Autodesk Inventor part; units mm, degrees
ref_plane "YZ Plane" through (0, 0, 0) normal (1, 0, 0) x (0, 1, 0)
ref_plane "XZ Plane" through (0, 0, 0) normal (0, 1, 0) x (-1, 0, 0)
ref_plane "XY Plane" through (0, 0, 0) normal (0, 0, 1) x (1, 0, 0)
sketch "Sketch1" plane through (0, 0, 0) normal (0, 0, 1) x (1, 0, 0)
  circle A0 centre (0, 91.8009) radius 38.1 construction
  circle A1 centre (0, -91.8009) radius 38.1 construction
  line L0 (0, 91.8009) -> (0, -91.8009) construction
  circle A2 centre (-25.4, 0) radius 57.15 construction
  circle A3 centre (0, 91.8009) radius 14.2875
  circle A4 centre (0, -91.8009) radius 14.2875
  circle A5 centre (0, -91.8009) radius 33.3375 construction
  circle A6 centre (0, 91.8009) radius 33.3375 construction
  circle A7 centre (-142.9967, -39.6875) radius 14.3256 construction
  circle A8 centre (0, -91.8009) radius 23.876 construction
  line L1 (-142.9967, -39.6875) -> (0, -91.8009) construction
  circle A9 centre (-142.9967, 39.6875) radius 14.3256 construction
  circle A10 centre (0, 91.8009) radius 23.876 construction
  line L2 (0, 91.8009) -> (-142.9967, 39.6875) construction
  circle A11 centre (-142.9967, 39.6875) radius 39.6875 construction
  circle A12 centre (-142.9967, -39.6875) radius 39.6875 construction
  line L3 (-142.9967, 39.6875) -> (-142.9967, -39.6875) construction
  line L4 (-138.9458, 25.9466) -> (6.7516, 68.8994) construction
  line L5 (-9.5669, 113.6764) -> (-148.7368, 52.8128) construction
  line L6 (-138.9458, -25.9466) -> (6.7516, -68.8994) construction
  circle A13 centre (-142.9967, 39.6875) radius 14.2875
  circle A14 centre (-142.9967, -39.6875) radius 14.2875
  circle A15 centre (-187.9418, -47.625) radius 5.9531 construction
  circle A16 centre (-187.9418, -47.625) radius 9.525
  circle A17 centre (-187.9418, -47.625) radius 17.4625 construction
  circle A18 centre (-187.9418, -47.625) radius 17.4625 construction
  circle A19 centre (-187.9418, -47.625) radius 17.4625 construction
  circle A20 centre (-187.9418, -47.625) radius 17.4625 construction
  circle A21 centre (-187.9418, -47.625) radius 17.4625 construction
  circle A22 centre (-19.05, 0) radius 57.15 construction
  circle A23 centre (-187.9418, -47.625) radius 19.05 construction
  line L7 (-241.3, 101.6) -> (-215.9, 101.6) construction
  line L8 (-215.9, 101.6) -> (-215.9, -101.6) construction
  line L9 (-215.9, -101.6) -> (-241.3, -101.6) construction
  line L10 (-241.3, -101.6) -> (-241.3, 101.6)
  line L11 (-142.9967, -39.6875) -> (-187.9418, -47.625) construction
  line L12 (-77.6563, 63.5) -> (-77.6563, -63.5) construction
  line L13 (-22.4906, -57.0463) -> (2.007, -58.5239)
  arc A24 (2.007, 58.5239) -> (27.142, 111.1581) centre (0, 91.8009) ccw
  arc A25 (-22.4906, 57.0463) -> (-22.4906, -57.0463) centre (-19.05, 0) ccw
  line L14 (2.007, 58.5239) -> (-22.4906, 57.0463)
  arc A26 (27.142, -111.1581) -> (2.007, -58.5239) centre (0, -91.8009) ccw
  arc A27 (3.8774, 143.7787) -> (-0.8591, 145.6978) centre (0, 141.0134) ccw
  circle A28 centre (0, 91.8009) radius 44.45 construction
  line L15 (3.8774, 143.7787) -> (27.142, 111.1581)
  line L16 (-0.8591, 145.6978) -> (-241.3, 101.6)
  arc A29 (-0.8591, -145.6978) -> (3.8774, -143.7787) centre (0, -141.0134) ccw
  line L17 (-241.3, -101.6) -> (-0.8591, -145.6978)
  line L18 (27.142, -111.1581) -> (3.8774, -143.7787)
  circle A30 centre (0, -91.8009) radius 44.45 construction
  line L19 (0, 112.8194) -> (0, 70.7824) construction
  line L20 (-142.9967, 60.706) -> (-142.9967, 18.669) construction
  line L21 (-142.9967, -18.669) -> (-142.9967, -60.706) construction
  line L22 (0, -70.7824) -> (0, -112.8194) construction
  line L23 (-228.6, 50.8) -> (-228.6, -50.8) construction
  line L24 (-187.9418, -15.875) -> (-187.9418, -79.375) construction
  circle A31 centre (-187.9418, -15.875) radius 4.7625 construction
  line L25 (-148.7368, -52.8128) -> (-9.5669, -113.6764) construction
  line L26 (-187.9418, -47.625) -> (-187.9418, -30.1625) construction
  circle A32 centre (-187.9418, -47.625) radius 17.4625 construction
  point P0 (0, 0)
  point P1 (0, 0)
  point P2 (-172.8189, -38.8937)
  point P3 (-203.0648, -38.8938)
  point P4 (-203.0648, -56.3562)
  point P5 (-187.9418, -65.0875)
  point P6 (-215.9, 0)
  point P7 (-228.6, 0)
  point P8 (-228.6, 0)
  point P9 (-228.6, 101.6)
  point P10 (-172.8189, -56.3562)
  dimension "d15" = 34.925
  dimension "d0" = 76.2
  dimension "d1" = 76.2
  dimension "d2" = 114.3
  dimension "d4" = 183.6018
  dimension "d5" = 28.575
  dimension "d6" = 19.05
  dimension "d7" = 28.6512
  dimension "d8" = 47.752
  dimension "d9" = 79.375
  dimension "d10" = 142.9967
  dimension "d11" = 152.1968
  dimension "d12" = 28.575
  dimension "d13" = 11.9062
  dimension "d14" = 19.05
  dimension "d18" = 360
  dimension "d20" = 6.35
  dimension "d21" = 38.1
  dimension "d22" = 25.4
  dimension "d23" = 203.2
  dimension "d24" = 241.3
  dimension "d26" = 127
  dimension "d29" = 9.525
  dimension "d30" = 6.35
  dimension "d32" = 42.037
  dimension "d33" = 42.037
  dimension "d34" = 42.037
  dimension "d35" = 42.037
  dimension "d36" = 25.4
  dimension "d44" = 101.6
  dimension "d45" = 63.5
  dimension "d47" = 9.525
  dimension "d49" = 53.975
extrude "Extrusion1" add sketch "Sketch1" along normal blind 6.35
hole "Hole1" at (-172.8189, -38.8937, 0) at (-187.9418, -30.1625, 0) at (-203.0648, -38.8938, 0) at (-203.0648, -56.3562, 0) at (-187.9418, -65.0875, 0) at (-77.6563, 63.5, 0) at (-77.6563, -63.5, 0) at (0, 112.8194, 0) at (0, 70.7824, 0) at (-142.9967, 60.706, 0) at (-142.9967, 18.669, 0) at (-142.9967, -18.669, 0) at (-142.9967, -60.706, 0) at (0, -70.7824, 0) at (0, -112.8194, 0) at (-228.6, 50.8, 0) at (-228.6, 0, 0) at (-228.6, -50.8, 0) at (-187.9418, -15.875, 0) at (-187.9418, -79.375, 0) at (0, 141.0134, 0) at (0, -141.0134, 0) at (-172.8189, -56.3562, 0) direction (0, 0, 1) diameter 5.1054 end through all
properties part number "GP6-001" material "Polycarbonate, Smoke"
CAD build for the part. Positions are in the model's coordinates, mm. A direction names the side the tool comes from. Give positions to 0.01 mm unless a question says otherwise; leave off trailing zeros. Loops run counter-clockwise (first coordinate to the right, second up) from the corner with the lowest first, then second, coordinate; pieces in that order, holes last. Notation, with made-up numbers: (46, -8) - (97, -8) arc R24 ccw to (97, 31) - close; hole circle Ø1 at (-6, -28). An arc over 180 degrees is marked (long way). Put each result on its own line as item: value.
Q1. Tool access for faces 5 (the face through (-10.07, 57.795, 3.131)), 6 (the face through (-119.396, 123.958, 3.131)): list every direction of +Z, -Z, +X, -X, +Y, -Y with a clear straight run to the whole face (end or side of a thin tool).
Filled in:
face 5: +Z, -Z, +X
face 6: +Z, -Z, -X, +Y
Q2. Mould opens along X. For faces 1 (the face through (-129.799, -34.215, 3.131)), 2 (the face through (-241.3, -1, 3)), 3 (the face through (-106, 2, 6.35)), 4 (the face through (-10.413, -57.775, 3.131)) say: pulls with the +X half, pulls with the -X half, needs draft (parallel to the pull), parting line crosses it, or undercut.
Filled in:
face 1: undercut
face 2: pulls with the -X half
face 3: needs draft
face 4: pulls with the +X half
Q3. Flat gauge pin, fed straight in: pin 1 (23 mm diameter, centred on x = 0, y = 91.8, fed in from -Z). Where does the tip first touch, or does it go through?
Filled in:
pin 1: passes through
Q4. Probe line 1 along Y through (x, z) = (-6.5, 3.5); line 2 along Y through (x, z) = (-227, 4.25); line 3 along Y through (x, z) = (-135, 0.5). List the from-to ranges inside material, lowest first.
Filled in:
line 1: y = -144.66 to -104.52, -79.08 to -58.01, 58.01 to 79.08, 104.52 to 144.66
line 2: y = -104.22 to -52.79, -48.81 to -1.99, 1.99 to 48.81, 52.79 to 104.22
line 3: y = -121.1 to -51.53, -27.85 to 27.85, 51.53 to 121.1
Q5. Slice it at A-A (x = -19.05). Give the cut face in (y, z).
Filled in:
outline: (-142.36, 0) - (-57.25, 0) - (-57.25, 6.35) - (-142.36, 6.35) - close; (57.25, 0) - (142.36, 0) - (142.36, 6.35) - (57.25, 6.35) - close
Q6. Slice it at C-C (z = 2.25). Give the number of separate pieces and of enclosed holes in the cut face, plus the area to 3 significant figures.
Filled in:
separate pieces: 1
enclosed holes: 28
area: 53,000 mm²
Q7. Slice it at B-B (y = 124.5). Give the cut face in (x, z), plus the area to 3 significant figures.
Filled in:
outline: (-116.44, 0) - (17.63, 0) - (17.63, 6.35) - (-116.44, 6.35) - close
area: 851 mm²
